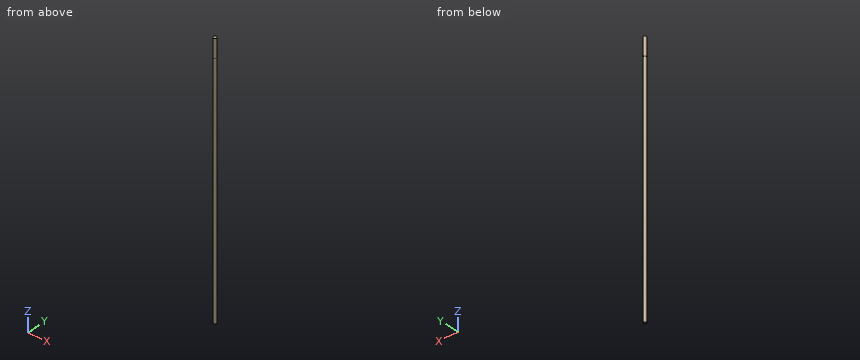
from build123d import *

# Parameters (mm, degrees)
SKETCH1_R           = 2.3495
SKETCH1_R_2         = 1.5625
BOSS_EXTRUDE1_DEPTH = 400.0000001
SKETCH2_R           = 2.75
BOSS_EXTRUDE2_DEPTH = 30


with BuildPart() as part:
    # Sketch1 → Boss-Extrude1 (new body)
    with BuildSketch(Plane.XY):
        with Locations(Location((0, 0, 0), (0, 0, 180))):
            Circle(SKETCH1_R)
        with Locations(Location((0, 0, 0), (0, 0, 180))):
            Circle(SKETCH1_R_2, mode=Mode.SUBTRACT)
    extrude(amount=BOSS_EXTRUDE1_DEPTH)

    # Sketch2 → Boss-Extrude2 (add)
    with BuildSketch(Plane.XY.offset(400.0000001)):
        Circle(SKETCH2_R)
    extrude(amount=BOSS_EXTRUDE2_DEPTH)


solid = part.part
Geometry check sheet. Reference: the model listing, model coordinates, mm. Give positions to 0.01 mm unless a question says otherwise; leave off trailing zeros. Loops run counter-clockwise (first coordinate to the right, second up) from the corner with the lowest first, then second, coordinate; pieces in that order, holes last.
(1) Thickness scan on L1, parallel to Y at x = 0, z = 83; L2, parallel to X at y = -0.25, z = 368; L3, parallel to Z at x = -0.5, y = -1.2. Record the ranges inside material, lowest first.
From the geometry:
L1: y = -2.35 to -1.56, 1.56 to 2.35
L2: x = -2.34 to -1.54, 1.54 to 2.34
L3: z = 400 to 430
(2) Section check A-A on x = 0. Record the cut outline in (y, z), then the cut area to 3 significant figures.
From the geometry:
outline: (-2.75, 400) - (-2.35, 400) - (-2.35, 0) - (-1.56, 0) - (-1.56, 400) - (1.56, 400) - (1.56, 0) - (2.35, 0) - (2.35, 400) - (2.75, 400) - (2.75, 430) - (-2.75, 430) - close
area: 795 mm2
(3) Section check C-C on z = 332.5. Record the cut outline in (x, y) (1 decimal).
From the geometry:
outline: circle Ø4.7 at (0, 0); hole circle Ø3.1 at (0, 0)
(4) Depth check by flat-ended pin: pin 1 Ø1.5 at (x, z) = (-1.5, 220.5) entering from -Y. Enter the tip coordinate at first touch or a pass-through.
From the geometry:
pin 1: stops at y = -2.23
